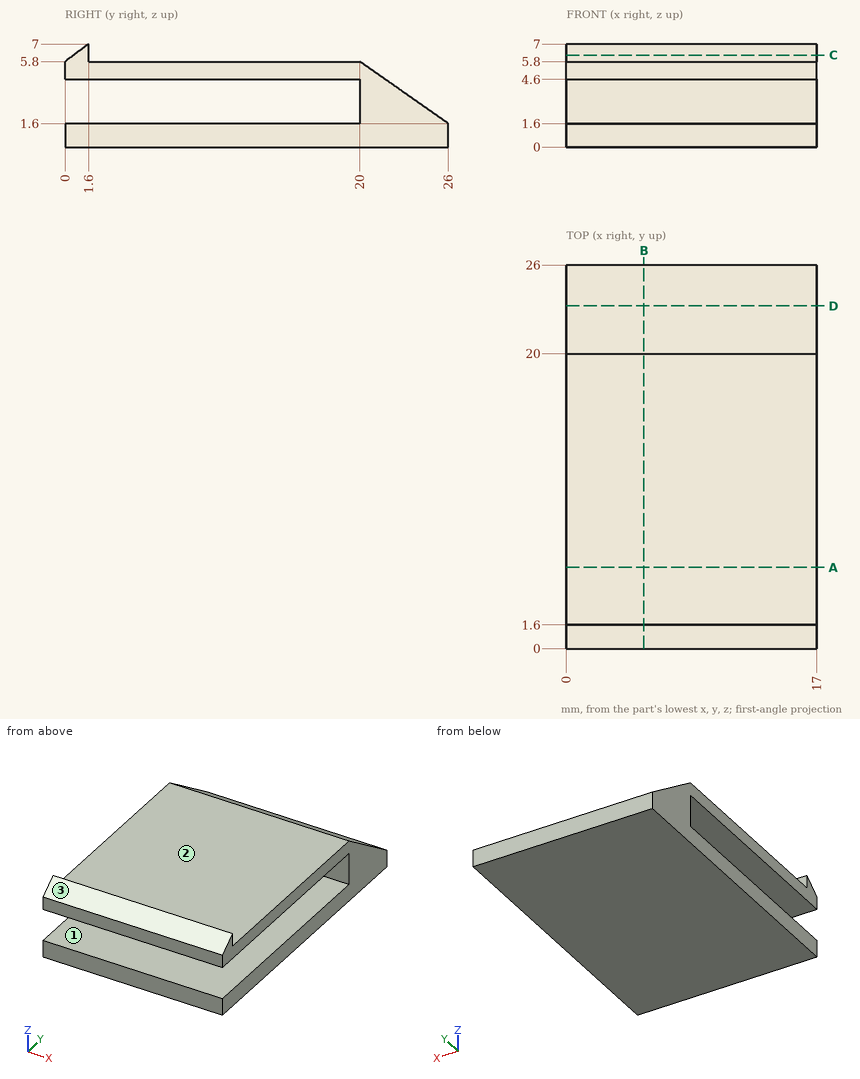
Input: dimensioned drawing with shaded views. Units: mm. Origin: part minimum x, y, z. A direction names the side the tool comes from. Give positions to 0.01 mm unless a question says otherwise; leave off trailing zeros. Write each loop counter-clockwise with the first axis right and the second up, starting at its lowest first coordinate (ties: lowest second). Pieces come first, ordered by that corner, then holes.
1. Section query D-D (y = 23.25). Return the cut outline in (x, z) (3 decimals).
2. Material intervals for line 1 along Z through (x, y) = (7, 7.5); line 2 along Y through (x, z) = (13.5, 6.5); line 3 along Z through (x, y) = (14.75, 23.25) (3 decimals), sorted ascending.
3. Access query for the marked faces 1, 2 and 3. Directions: +Z, -Z, +X, -X, +Y, -Y. A direction counts if a zero-diameter tool reaches every point of the face in a straight line with its end or side. Return the directions, or none.
4. First-contact query: pin 1 (1 mm diameter, centred on y = 3.5, z = 6, fed in from -X); pin 2 (1 mm diameter, centred on x = 10.5, z = 6.5, fed in from +Y); pin 3 (4 mm diameter, centred on x = 5.5, z = 6, fed in from +Y); pin 4 (8.5 mm diameter, centred on x = 9.5, y = 14.5, fed in from +Z). Flat tips, straight axial feed; report the tip coordinate or a pass-through.
5. Section query C-C (z = 6.25). Return the cut outline in (x, y).
6. Section query B-B (x = 5.25). Return the cut outline in (y, z), then the cut area to 3 significant figures.
7. Section query A-A (y = 5.5). Return the cut outline in (x, z).
Output values:
1. outline: (0, 0) - (17, 0) - (17, 3.525) - (0, 3.525) - close
2. line 1: z = 0 to 1.6, 4.6 to 5.8
2. line 2: y = 0.93 to 1.6
2. line 3: z = 0 to 3.525
3. face 1: +X, -X, -Y
3. face 2: +Z, +X, -X, +Y
3. face 3: +Z, +X, -X, -Y
4. pin 1: stops at x = 0
4. pin 2: stops at y = 1.6
4. pin 3: stops at y = 22.57
4. pin 4: stops at z = 5.8
5. outline: (0, 0.6) - (17, 0.6) - (17, 1.6) - (0, 1.6) - close
6. outline: (0, 0) - (26, 0) - (26, 1.6) - (20, 5.8) - (1.6, 5.8) - (1.6, 7) - (0, 5.8) - (0, 4.6) - (20, 4.6) - (20, 1.6) - (0, 1.6) - close
6. area: 79.2 mm2
7. outline: (0, 0) - (17, 0) - (17, 1.6) - (0, 1.6) - close; (0, 4.6) - (17, 4.6) - (17, 5.8) - (0, 5.8) - close
